from build123d import *

# Parameters (mm, degrees)
SKETCH_2_R          = 12
SKETCH_2_R_2        = 10.5
SKETCH_2_R_3        = 4
SKETCH_2_R_4        = 2
BOSS_EXTRUDE1_DEPTH = 6


with BuildPart() as part:
    # 草图2 → Boss-Extrude1 (new body)
    # profile 1 of 6: a face of its own
    with BuildSketch(Plane(origin=(0, 0, 0), x_dir=(0, 0, -1), z_dir=(1, 0, 0))):
        Circle(SKETCH_2_R)
        Circle(SKETCH_2_R_2, mode=Mode.SUBTRACT)
    # profile 2 of 6: a face of its own
    with BuildSketch(Plane(origin=(0, 0, 0), x_dir=(0, 0, -1), z_dir=(1, 0, 0))):
        with BuildLine():
            Line((-0.741872063, 10.473758917), (-0.282617929, 3.990003397))
            ThreePointArc((-0.282617929, 3.990003397), (0.501223543, 3.968472623), (1.265803275, 3.794435672))
            Line((1.265803275, 3.794435672), (3.322733597, 9.960393639))
            ThreePointArc((3.322733597, 9.960393639), (1.315711801, 10.417240635), (-0.741872063, 10.473758917))
        make_face()
    # profile 3 of 6: a face of its own
    with BuildSketch(Plane(origin=(0, 0, 0), x_dir=(0, 0, -1), z_dir=(1, 0, 0))):
        with BuildLine():
            Line((10.473758917, 0.741872063), (3.990003397, 0.282617929))
            ThreePointArc((3.990003397, 0.282617929), (3.997500068, 0.141397335), (4, 0))
            ThreePointArc((4, 0), (3.948274477, -0.64119315), (3.794435672, -1.265803275))
            Line((3.794435672, -1.265803275), (9.960393639, -3.322733597))
            ThreePointArc((9.960393639, -3.322733597), (10.364220502, -1.68313202), (10.5, 0))
            ThreePointArc((10.5, 0), (10.493437678, 0.371168005), (10.473758917, 0.741872063))
        make_face()
    # profile 4 of 6: a face of its own
    with BuildSketch(Plane(origin=(0, 0, 0), x_dir=(0, 0, -1), z_dir=(1, 0, 0))):
        with BuildLine():
            ThreePointArc((0.282617929, -3.990003397), (-0.501223543, -3.968472623), (-1.265803275, -3.794435672))
            Line((-1.265803275, -3.794435672), (-3.322733597, -9.960393639))
            ThreePointArc((-3.322733597, -9.960393639), (-1.315711801, -10.417240635), (0.741872063, -10.473758917))
            Line((0.741872063, -10.473758917), (0.282617929, -3.990003397))
        make_face()
    # profile 5 of 6: a face of its own
    with BuildSketch(Plane(origin=(0, 0, 0), x_dir=(0, 0, -1), z_dir=(1, 0, 0))):
        Circle(SKETCH_2_R_3)
        Circle(SKETCH_2_R_4, mode=Mode.SUBTRACT)
    # profile 6 of 6: a face of its own
    with BuildSketch(Plane(origin=(0, 0, 0), x_dir=(0, 0, -1), z_dir=(1, 0, 0))):
        with BuildLine():
            ThreePointArc((-3.990003397, -0.282617929), (-3.968472623, 0.501223543), (-3.794435672, 1.265803275))
            Line((-3.794435672, 1.265803275), (-9.960393639, 3.322733597))
            ThreePointArc((-9.960393639, 3.322733597), (-10.417240635, 1.315711801), (-10.473758917, -0.741872063))
            Line((-10.473758917, -0.741872063), (-3.990003397, -0.282617929))
        make_face()
    extrude(amount=BOSS_EXTRUDE1_DEPTH)


solid = part.part
Here's how the part is built. I have some questions about the finished solid (model axes, mm). A direction names the side the tool comes from. Round coordinates to 2 decimals unless told otherwise and drop trailing zeros. Loops run counter-clockwise (first coordinate to the right, second up) from the corner with the lowest first, then second, coordinate; pieces in that order, holes last. Notation, with made-up numbers: (18.25, 39.5) - (66.25, 39.5) arc R30 cw to (66.25, 64.5) - close; hole circle Ø3 at (11.25, 26). An arc over 180 degrees is marked (long way). One line per question, with ' | ' between items. Start each with the question number.
Q1. I want a section at B-B (y = -5.25). Write out the boundary of the cut face in (x, z).
Q2. I want a section at C-C (x = 2.7). Write out the boundary of the cut face in (y, z), then the cut area to 3 significant figures.
Q3. I want a section at A-A (z = 0). Write out the boundary of the cut face in (x, y), then the cut area to 3 significant figures.
Q4. We'd pull the mould along Z, two halves only. Please class faces 3 (the cylindrical face through (2.96, 0.53, 11.99)), 4 (the flat face through (6, 0.2, -2.5)), 5 (the cylindrical face through (3, -2.4, 3.2)): +Z half, -Z half, draft (parallel to the pull), parting line (faces both ways), or undercut.
Q5. Will these pins go through, and if not, where does the flat tip stop? pin 1 (3 mm diameter, centred on x = 5.5, z = 8.5, fed in from +Y); pin 2 (2 mm diameter, centred on x = 3, y = -9, fed in from +Z); pin 3 (2 mm diameter, centred on x = 2.5, z = 9, fed in from -Y).
Q6. For faces 1 (the flat face through (0, 0.2, -2.5)), 2 (the cylindrical face through (3, -3.2, -2.4)), which set-ups out of +Z, -Z, +X, -X, +Y, -Y let a thin tool reach every point of the face, with its end or its side?
Q7. Please list where these lines run through material, in increasing order: line 1 (Y direction, x = 4.45, z = 0); line 2 (Z direction, x = 2.2, y = -5); line 3 (Z direction, x = 3.95, y = -6.5). Write a range as [from, to].
Response values:
1) outline: (0, -10.79) - (6, -10.79) - (6, -9.09) - (0, -9.09) - close; (0, -0.37) - (6, -0.37) - (6, 1.75) - (0, 1.75) - close; (0, 9.09) - (6, 9.09) - (6, 10.79) - (0, 10.79) - close
2) outline: circle Ø24 at (0, 0); hole (-10.47, -0.74) arc R10.5 ccw to (-3.32, -9.96) - (-1.27, -3.79) arc R4 cw to (-3.99, -0.28) - close; hole (-9.96, 3.32) - (-3.79, 1.27) arc R4 cw to (-0.28, 3.99) - (-0.74, 10.47) arc R10.5 ccw to start; hole circle Ø4 at (0, 0); hole (0.28, -3.99) - (0.74, -10.47) arc R10.5 ccw to (9.96, -3.32) - (3.79, -1.27) arc R4 cw to start; hole (1.27, 3.79) arc R4 cw to (3.99, 0.28) - (10.47, 0.74) arc R10.5 ccw to (3.32, 9.96) - close | area: 218 mm²
3) outline: (0, -12) - (6, -12) - (6, -2) - (0, -2) - close; (0, 2) - (6, 2) - (6, 12) - (0, 12) - close | area: 120 mm²
4) face 3: parting line | face 4: draft | face 5: undercut
5) pin 1: stops at y = 9.75 | pin 2: stops at z = 8.94 | pin 3: stops at y = -8.94
6) face 1: +Z, -Z, -X, +Y, -Y | face 2: +X, -X
7) line 1: y = [-12, -2], [2, 12] | line 2: z = [-10.91, -9.23], [-0.35, 1.67], [9.23, 10.91] | line 3: z = [-10.09, -8.25], [-0.46, 2.17], [8.25, 10.09]
